Can you work these out from the model? Positions are in its coordinate system, mm. Face numbers are marked on the shaded views. A direction names the side the tool comes from. Coordinates: 2 decimals unless noted, no trailing zeros. Loops run counter-clockwise (first coordinate to the right, second up) from the corner with the lowest first, then second, coordinate; pieces in that order, holes last. Notation, with made-up numbers: (62, 33.25) -> (74, 33.25) arc R14 cw to (74, 50.25) -> close; hole circle Ø4 at (6, 5). An arc over 180 degrees is marked (long way). Put each result on its own line as item: value. Start each with the question number.
Item 1: If we section it at D-D on x = 2.5: Please give me the cut outline in (y, z).
Item 2: For the marked faces 1, 2 and 3, which set-ups out of +Z, -Z, +X, -X, +Y, -Y let a thin tool reach every point of the face, with its end or its side?
Item 3: Please list where these lines run through material, in increasing order: L1, parallel to Y at x = 0, z = 5.45 (3 decimals); L2, parallel to X at y = 15.2, z = 0 (3 decimals); L3, parallel to Y at x = 2, z = -0.5. Write a range as from..to.
Item 4: We'd pull the mould along X, two halves only. Please class the marked faces 4, 5 and 6: pulls with the +X half, pulls with the -X half, needs draft (parallel to the pull), parting line crosses it, or undercut.
Item 5: Will these pins go through, and if not, where does the flat tip stop? P1, Ø1.4, axis at x = 0, y = 15, coming from the +Z side; P2, Ø1.2, axis at x = -0.5, y = 7.5, coming from the +Z side; P3, Ø0.5, axis at y = 14, z = 2, coming from the -X side.
Item 6: If we section it at B-B on y = 12.25: Please give me the cut outline in (x, z) (3 decimals), plus the area to 3 significant figures.
Item 7: If we section it at A-A on z = 0: Please give me the cut outline in (x, y) (3 decimals).
Item 8: If we section it at C-C on y = 7.75: Please give me the cut outline in (x, z).
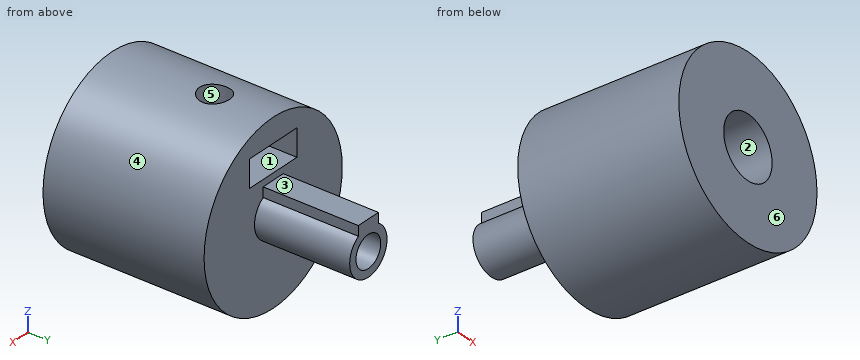
```python
from build123d import *

# Parameters (mm, degrees)
SKETCH1_R           = 6
BOSS_EXTRUDE1_DEPTH = 10
SKETCH2_R           = 1.025
CUT_EXTRUDE1_DEPTH  = 7
SKETCH4_R           = 2.1
CUT_EXTRUDE4_DEPTH  = 11.0000001
SKETCH5_W           = 0.95
SKETCH5_H           = 7.069146706
BOSS_EXTRUDE2_DEPTH = 1.2
SKETCH7_R           = 6
BOSS_EXTRUDE3_DEPTH = 1
SKETCH8_R           = 1.62
SKETCH8_W           = 1.74
SKETCH8_H           = 0.84
BOSS_EXTRUDE4_DEPTH = 6.5
SKETCH9_R           = 1.075
CUT_EXTRUDE5_DEPTH  = 6
CUT_EXTRUDE2_START  = 2.5
CUT_EXTRUDE2_DEPTH  = 1.85


with BuildPart() as part:
    # Sketch1 → Boss-Extrude1 (new body)
    with BuildSketch(Plane(origin=(0, 0, 0), x_dir=(1, 0, 0), z_dir=(0, 1, 0))):
        Circle(SKETCH1_R)
    extrude(amount=BOSS_EXTRUDE1_DEPTH)

    # Sketch2 → Cut-Extrude1 (cut, through all)
    with BuildSketch(Plane.XY):
        with Locations((0, 7)):
            Circle(SKETCH2_R)
    extrude(amount=CUT_EXTRUDE1_DEPTH, mode=Mode.SUBTRACT)

    # Sketch4 → Cut-Extrude4 (cut, through all)
    with BuildSketch(Plane(origin=(0, 0, 0), x_dir=(1, 0, 0), z_dir=(0, 1, 0))):
        Circle(SKETCH4_R)
    extrude(amount=CUT_EXTRUDE4_DEPTH, mode=Mode.SUBTRACT)

    # Sketch5 → Boss-Extrude2 (add)
    with BuildSketch(Plane(origin=(0, 10, 0), x_dir=(1, 0, 0), z_dir=(0, 1, 0))):
        Rectangle(SKETCH5_W, SKETCH5_H)
    extrude(amount=-BOSS_EXTRUDE2_DEPTH)

    # Sketch7 → Boss-Extrude3 (add)
    with BuildSketch(Plane(origin=(0, 10, 0), x_dir=(1, 0, 0), z_dir=(0, 1, 0))):
        Circle(SKETCH7_R)
    extrude(amount=BOSS_EXTRUDE3_DEPTH)

    # Sketch8 → Boss-Extrude4 (add)
    with BuildSketch(Plane(origin=(0, 11, 0), x_dir=(1, 0, 0), z_dir=(0, 1, 0))):
        Circle(SKETCH8_R)
        with Locations((0, -1.62)):
            Rectangle(SKETCH8_W, SKETCH8_H)
    extrude(amount=BOSS_EXTRUDE4_DEPTH)

    # Sketch9 → Cut-Extrude5 (cut)
    with BuildSketch(Plane(origin=(0, 17.5, 0), x_dir=(1, 0, 0), z_dir=(0, 1, 0))):
        Circle(SKETCH9_R)
    extrude(amount=-CUT_EXTRUDE5_DEPTH, mode=Mode.SUBTRACT)

    # Sketch3 → Cut-Extrude2 (cut)
    with BuildSketch(Plane.XY.offset(CUT_EXTRUDE2_START)):
        Polygon((0, 4.621316891), (2.06, 5.810658445), (2.06, 8.189341555), (2.06, 11.363105915), (-2.06, 11.363105915), (-2.06, 8.189341555), (-2.06, 5.810658445), align=None)
    extrude(amount=CUT_EXTRUDE2_DEPTH, mode=Mode.SUBTRACT)


solid = part.part
```
Solutions:
1. outline: (0, -5.45) -> (11, -5.45) -> (11, 5.45) -> (0, 5.45) -> close
2. face 1: +Y
2. face 2: -Y
2. face 3: +Z, +X, -X, +Y
3. L1: 0..5.975, 8.025..11
3. L2: -1.62..-1.075, 1.075..1.62
3. L3: 10..11
4. face 4: parting line crosses it
4. face 5: undercut
4. face 6: needs draft
5. P1: z = 2.04
5. P2: z = 6
5. P3: x = -0.87
6. outline: (-0.87, 1.367) arc R1.62 ccw (long way) to (0.87, 1.367) -> (0.87, 2.04) -> (-0.87, 2.04) -> close; hole circle Ø2.15 at (0, 0)
6. area: 5.49 mm^2
7. outline: (-6, 0) -> (-2.1, 0) -> (-2.1, 10) -> (-0.475, 10) -> (-0.475, 8.8) -> (0.475, 8.8) -> (0.475, 10) -> (2.1, 10) -> (2.1, 0) -> (6, 0) -> (6, 11) -> (1.62, 11) -> (1.62, 17.5) -> (1.075, 17.5) -> (1.075, 11.5) -> (-1.075, 11.5) -> (-1.075, 17.5) -> (-1.62, 17.5) -> (-1.62, 11) -> (-6, 11) -> close
8. outline: (-2.06, 2.5) -> (-2.06, 4.35) -> (-0.7, 4.35) -> (-0.7, 5.96) arc R6 ccw (long way) to (0.7, 5.96) -> (0.7, 4.35) -> (2.06, 4.35) -> (2.06, 2.5) -> (0.7, 2.5) -> (0.7, 1.98) arc R2.1 cw (long way) to (-0.7, 1.98) -> (-0.7, 2.5) -> close
